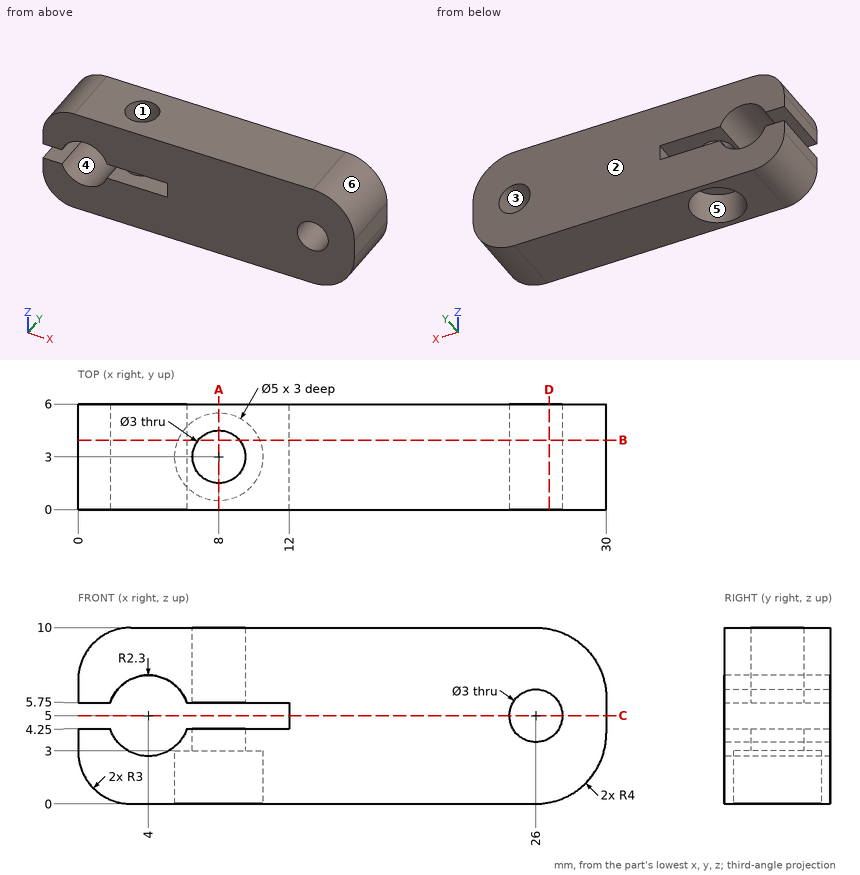
Job drawing, mm, ordinate dimensions from the low corner. One solid piece. A direction names the side the tool comes from. Round coordinates to 2 decimals unless told otherwise and drop trailing zeros. Loops run counter-clockwise (first coordinate to the right, second up) from the corner with the lowest first, then second, coordinate; pieces in that order, holes last.
(1) Wall check: line 1 along Z through (x, y) = (11.75, 0.5); line 2 along X through (y, z) = (2, 6.25); line 3 along Z through (x, y) = (6.25, 1.8). Give the ranges that are in metal, low to high.
(2) Two-plate mould, pull along Y, no slides. Class the marked faces 1, 2 and 3: +Y half, -Y half, draft (parallel to the pull), parting line (faces both ways), or undercut.
(3) Cut at B-B (y = 3.95). State how many separate pieces and enclosed holes the cut face has, plus the area to 3 significant figures.
(4) Cut at D-D (x = 26.75). Give the cut face in (y, z).
(5) Cut at C-C (z = 5). Give the cut face in (x, y), plus the area to 3 significant figures.
(6) Drop flat-ended pins along their axis: pin 1 (2.5 mm diameter, centred on x = 8, y = 3, fed in from +Z); pin 2 (1.5 mm diameter, centred on x = 0.5, y = 2, fed in from -Z); pin 3 (2 mm diameter, centred on x = 1, y = 3, fed in from +Z); pin 4 (1 mm diameter, centred on y = 2, z = 9, fed in from -X). Give the stop position or say it passes through.
(7) Which spindle directions (+Z, -Z, +X, -X, +Y, -Y) get a long thin tool onto all of the face, cutting with end or side? Do the marked faces 4, 5 and 6. Say none if no direction does.
(8) Cut at A-A (x = 8). Give the cut face in (y, z).
Findings below:
1. line 1: z = 0 to 4.25, 5.75 to 10
1. line 2: x = 0 to 2.07, 5.93 to 6.88, 9.12 to 25.17, 26.83 to 29.99
1. line 3: z = 3 to 4.25, 5.75 to 10
2. face 1: undercut
2. face 2: +Y half
2. face 3: draft
3. separate pieces: 3
3. enclosed holes: 1
3. area: 228 mm2
4. outline: (0, 0.07) - (6, 0.07) - (6, 3.7) - (0, 3.7) - close; (0, 6.3) - (6, 6.3) - (6, 9.93) - (0, 9.93) - close
5. outline: (12, 0) - (24.5, 0) - (24.5, 6) - (12, 6) - close; (27.5, 0) - (30, 0) - (30, 6) - (27.5, 6) - close
5. area: 90.0 mm2
6. pin 1: passes through
6. pin 2: stops at z = 0.56
6. pin 3: stops at z = 9.83
6. pin 4: stops at x = 0.4
7. face 4: +Y, -Y
7. face 5: -Z
7. face 6: +Z, +X, +Y, -Y
8. outline: (0, 0) - (0.5, 0) - (0.5, 3) - (1.5, 3) - (1.5, 4.25) - (0, 4.25) - close; (0, 5.75) - (1.5, 5.75) - (1.5, 10) - (0, 10) - close; (4.5, 3) - (5.5, 3) - (5.5, 0) - (6, 0) - (6, 4.25) - (4.5, 4.25) - close; (4.5, 5.75) - (6, 5.75) - (6, 10) - (4.5, 10) - close
